from build123d import *
from OCP.BRepFilletAPI import BRepFilletAPI_MakeChamfer

# Parameters (mm, degrees)
BOSS_EXTRUDE1_DEPTH = 5
BOSS_EXTRUDE2_DEPTH = 2
SKETCH5_W           = 2.803061543
SKETCH5_H           = 5
BOSS_EXTRUDE3_DEPTH = 1
BOSS_EXTRUDE4_DEPTH = 0.5
SKETCH7_W           = 5
SKETCH7_H           = 38
CHAMFER1_SIZE       = 0.3
CHAMFER1_SIZE2      = 0.173205081


with BuildPart() as part:
    # Sketch2 → Boss-Extrude1 (new, symmetric)
    with BuildSketch(Plane.XY):
        with BuildLine():
            Line((-14.696938457, 34.5), (-14.696938457, 9.5))
            ThreePointArc((-14.696938457, 9.5), (-16.784612343, 4.952452777), (-17.5, 0))
            Line((-17.5, 0), (-40, 0))
            ThreePointArc((-40, 0), (-35.043919369, 19.285323831), (-21.403814237, 33.791666667))
            Line((-21.403814237, 33.791666667), (-21.403814237, 30.791666667))
            ThreePointArc((-21.403814237, 30.791666667), (-18.145358092, 32.817616911), (-14.696938457, 34.5))
        make_face()
    extrude(amount=BOSS_EXTRUDE1_DEPTH, both=True)

    # Sketch4 → Boss-Extrude2 (add)
    with BuildSketch(Plane.XY.offset(5)):
        Polygon((-17.5, 15), (-20, 14), (-20, 11), (-17.5, 10), (-17.5, 7), (-20, 6), (-20, 3), (-17.5, 2), (-17.5, 0), (-32.5, 0), (-32.5, 6.5), (-29.25, 9), (-29.25, 13), (-26, 15.5), (-26, 22), (-17.5, 22), align=None)
    extrude(amount=BOSS_EXTRUDE2_DEPTH)

    # Sketch5 → Boss-Extrude3 (add)
    with BuildSketch(Plane.XY.offset(5)):
        with Locations((-16.098469229, 17.5)):
            Rectangle(SKETCH5_W, SKETCH5_H)
    extrude(amount=BOSS_EXTRUDE3_DEPTH)

    # Sketch6 → Boss-Extrude4 (add)
    with BuildSketch(Plane.XY.offset(5)):
        Polygon((-26, 22), (-18.5, 26.5), (-17.5, 26.5), (-17.5, 22), align=None)
    extrude(amount=BOSS_EXTRUDE4_DEPTH)

    # Sketch7 → Cut-Revolve1 (revolve, cut)
    with BuildSketch(Plane(origin=(0, 0, 0), x_dir=(0, 0, -1), z_dir=(1, 0, 0))):
        with Locations((0, 19)):
            Rectangle(SKETCH7_W, SKETCH7_H)
    revolve(axis=Axis((0, 0, 2.5), (0, 0, -1)), mode=Mode.SUBTRACT)

    # Mirror1: part across plane


with BuildPart() as part_1:
    add(part.part)
    add(part.part.mirror(Plane.ZX))

    # Chamfer1: one chamfer whose edges measure the first distance from different faces: ONE call of the kernel's chamfer builder (chamfer() names one face for all edges)
    chamfer1_edges_1 = [part_1.edges().sort_by_distance(p)[0] for p in [
        (-17.5, -18.5, 7),
    ]]
    chamfer1_side_1 = [part_1.faces().sort_by_distance(p)[0] for p in [
        (-17.5, -20.094444444, 6.072222222),
    ]]
    chamfer1_edges_2 = [part_1.edges().sort_by_distance(p)[0] for p in [
        (-18.75, -2.5, 7),
    ]]
    chamfer1_side_2 = [part_1.faces().sort_by_distance(p)[0] for p in [
        (-18.75, -2.5, 6),
    ]]
    chamfer1_edges_3 = [part_1.edges().sort_by_distance(p)[0] for p in [
        (-20, -4.5, 7),
    ]]
    chamfer1_side_3 = [part_1.faces().sort_by_distance(p)[0] for p in [
        (-20, -4.5, 6),
    ]]
    chamfer1_edges_4 = [part_1.edges().sort_by_distance(p)[0] for p in [
        (-18.75, -6.5, 7),
    ]]
    chamfer1_side_4 = [part_1.faces().sort_by_distance(p)[0] for p in [
        (-18.75, -6.5, 6),
    ]]
    chamfer1_edges_5 = [part_1.edges().sort_by_distance(p)[0] for p in [
        (-17.5, -8.5, 7),
    ]]
    chamfer1_side_5 = [part_1.faces().sort_by_distance(p)[0] for p in [
        (-17.5, -8.5, 6),
    ]]
    chamfer1_edges_6 = [part_1.edges().sort_by_distance(p)[0] for p in [
        (-18.75, -10.5, 7),
    ]]
    chamfer1_side_6 = [part_1.faces().sort_by_distance(p)[0] for p in [
        (-18.75, -10.5, 6),
    ]]
    chamfer1_edges_7 = [part_1.edges().sort_by_distance(p)[0] for p in [
        (-20, -12.5, 7),
    ]]
    chamfer1_side_7 = [part_1.faces().sort_by_distance(p)[0] for p in [
        (-20, -12.5, 6),
    ]]
    chamfer1_edges_8 = [part_1.edges().sort_by_distance(p)[0] for p in [
        (-18.75, -14.5, 7),
    ]]
    chamfer1_side_8 = [part_1.faces().sort_by_distance(p)[0] for p in [
        (-18.75, -14.5, 6),
    ]]
    chamfer1_edges_9 = [part_1.edges().sort_by_distance(p)[0] for p in [
        (-21.75, -22, 7),
    ]]
    chamfer1_side_9 = [part_1.faces().sort_by_distance(p)[0] for p in [
        (-21.75, -22, 6.25),
    ]]
    chamfer1_edges_10 = [part_1.edges().sort_by_distance(p)[0] for p in [
        (-26, -18.75, 7),
    ]]
    chamfer1_side_10 = [part_1.faces().sort_by_distance(p)[0] for p in [
        (-26, -18.75, 6),
    ]]
    chamfer1_edges_11 = [part_1.edges().sort_by_distance(p)[0] for p in [
        (-27.625, -14.25, 7),
    ]]
    chamfer1_side_11 = [part_1.faces().sort_by_distance(p)[0] for p in [
        (-27.625, -14.25, 6),
    ]]
    chamfer1_edges_12 = [part_1.edges().sort_by_distance(p)[0] for p in [
        (-29.25, -11, 7),
    ]]
    chamfer1_side_12 = [part_1.faces().sort_by_distance(p)[0] for p in [
        (-29.25, -11, 6),
    ]]
    chamfer1_edges_13 = [part_1.edges().sort_by_distance(p)[0] for p in [
        (-30.875, -7.75, 7),
    ]]
    chamfer1_side_13 = [part_1.faces().sort_by_distance(p)[0] for p in [
        (-30.875, -7.75, 6),
    ]]
    chamfer1_edges_14 = [part_1.edges().sort_by_distance(p)[0] for p in [
        (-17.5, 0, 7),
    ]]
    chamfer1_side_14 = [part_1.faces().sort_by_distance(p)[0] for p in [
        (-17.5, 0, 6),
    ]]
    chamfer1_edges_15 = [part_1.edges().sort_by_distance(p)[0] for p in [
        (-18.75, 2.5, 7),
    ]]
    chamfer1_side_15 = [part_1.faces().sort_by_distance(p)[0] for p in [
        (-18.75, 2.5, 6),
    ]]
    chamfer1_edges_16 = [part_1.edges().sort_by_distance(p)[0] for p in [
        (-20, 4.5, 7),
    ]]
    chamfer1_side_16 = [part_1.faces().sort_by_distance(p)[0] for p in [
        (-20, 4.5, 6),
    ]]
    chamfer1_edges_17 = [part_1.edges().sort_by_distance(p)[0] for p in [
        (-18.75, 6.5, 7),
    ]]
    chamfer1_side_17 = [part_1.faces().sort_by_distance(p)[0] for p in [
        (-18.75, 6.5, 6),
    ]]
    chamfer1_edges_18 = [part_1.edges().sort_by_distance(p)[0] for p in [
        (-17.5, 8.5, 7),
    ]]
    chamfer1_side_18 = [part_1.faces().sort_by_distance(p)[0] for p in [
        (-17.5, 8.5, 6),
    ]]
    chamfer1_edges_19 = [part_1.edges().sort_by_distance(p)[0] for p in [
        (-18.75, 10.5, 7),
    ]]
    chamfer1_side_19 = [part_1.faces().sort_by_distance(p)[0] for p in [
        (-18.75, 10.5, 6),
    ]]
    chamfer1_edges_20 = [part_1.edges().sort_by_distance(p)[0] for p in [
        (-20, 12.5, 7),
    ]]
    chamfer1_side_20 = [part_1.faces().sort_by_distance(p)[0] for p in [
        (-20, 12.5, 6),
    ]]
    chamfer1_edges_21 = [part_1.edges().sort_by_distance(p)[0] for p in [
        (-18.75, 14.5, 7),
    ]]
    chamfer1_side_21 = [part_1.faces().sort_by_distance(p)[0] for p in [
        (-18.75, 14.5, 6),
    ]]
    chamfer1_edges_22 = [part_1.edges().sort_by_distance(p)[0] for p in [
        (-17.5, 18.5, 7),
    ]]
    chamfer1_side_22 = [part_1.faces().sort_by_distance(p)[0] for p in [
        (-17.5, 20.094444444, 6.072222222),
    ]]
    chamfer1_edges_23 = [part_1.edges().sort_by_distance(p)[0] for p in [
        (-21.75, 22, 7),
    ]]
    chamfer1_side_23 = [part_1.faces().sort_by_distance(p)[0] for p in [
        (-21.75, 22, 6.25),
    ]]
    chamfer1_edges_24 = [part_1.edges().sort_by_distance(p)[0] for p in [
        (-26, 18.75, 7),
    ]]
    chamfer1_side_24 = [part_1.faces().sort_by_distance(p)[0] for p in [
        (-26, 18.75, 6),
    ]]
    chamfer1_edges_25 = [part_1.edges().sort_by_distance(p)[0] for p in [
        (-27.625, 14.25, 7),
    ]]
    chamfer1_side_25 = [part_1.faces().sort_by_distance(p)[0] for p in [
        (-27.625, 14.25, 6),
    ]]
    chamfer1_edges_26 = [part_1.edges().sort_by_distance(p)[0] for p in [
        (-29.25, 11, 7),
    ]]
    chamfer1_side_26 = [part_1.faces().sort_by_distance(p)[0] for p in [
        (-29.25, 11, 6),
    ]]
    chamfer1_edges_27 = [part_1.edges().sort_by_distance(p)[0] for p in [
        (-30.875, 7.75, 7),
    ]]
    chamfer1_side_27 = [part_1.faces().sort_by_distance(p)[0] for p in [
        (-30.875, 7.75, 6),
    ]]
    chamfer1_edges_28 = [part_1.edges().sort_by_distance(p)[0] for p in [
        (-32.5, 0, 7),
    ]]
    chamfer1_side_28 = [part_1.faces().sort_by_distance(p)[0] for p in [
        (-32.5, 0, 6),
    ]]
    chamfer1 = BRepFilletAPI_MakeChamfer(part_1.part.solid().wrapped)
    for e in chamfer1_edges_1:
        chamfer1.Add(CHAMFER1_SIZE, CHAMFER1_SIZE2, e.wrapped, chamfer1_side_1[0].wrapped)  # the first distance lies on this face
    for e in chamfer1_edges_2:
        chamfer1.Add(CHAMFER1_SIZE, CHAMFER1_SIZE2, e.wrapped, chamfer1_side_2[0].wrapped)  # the first distance lies on this face
    for e in chamfer1_edges_3:
        chamfer1.Add(CHAMFER1_SIZE, CHAMFER1_SIZE2, e.wrapped, chamfer1_side_3[0].wrapped)  # the first distance lies on this face
    for e in chamfer1_edges_4:
        chamfer1.Add(CHAMFER1_SIZE, CHAMFER1_SIZE2, e.wrapped, chamfer1_side_4[0].wrapped)  # the first distance lies on this face
    for e in chamfer1_edges_5:
        chamfer1.Add(CHAMFER1_SIZE, CHAMFER1_SIZE2, e.wrapped, chamfer1_side_5[0].wrapped)  # the first distance lies on this face
    for e in chamfer1_edges_6:
        chamfer1.Add(CHAMFER1_SIZE, CHAMFER1_SIZE2, e.wrapped, chamfer1_side_6[0].wrapped)  # the first distance lies on this face
    for e in chamfer1_edges_7:
        chamfer1.Add(CHAMFER1_SIZE, CHAMFER1_SIZE2, e.wrapped, chamfer1_side_7[0].wrapped)  # the first distance lies on this face
    for e in chamfer1_edges_8:
        chamfer1.Add(CHAMFER1_SIZE, CHAMFER1_SIZE2, e.wrapped, chamfer1_side_8[0].wrapped)  # the first distance lies on this face
    for e in chamfer1_edges_9:
        chamfer1.Add(CHAMFER1_SIZE, CHAMFER1_SIZE2, e.wrapped, chamfer1_side_9[0].wrapped)  # the first distance lies on this face
    for e in chamfer1_edges_10:
        chamfer1.Add(CHAMFER1_SIZE, CHAMFER1_SIZE2, e.wrapped, chamfer1_side_10[0].wrapped)  # the first distance lies on this face
    for e in chamfer1_edges_11:
        chamfer1.Add(CHAMFER1_SIZE, CHAMFER1_SIZE2, e.wrapped, chamfer1_side_11[0].wrapped)  # the first distance lies on this face
    for e in chamfer1_edges_12:
        chamfer1.Add(CHAMFER1_SIZE, CHAMFER1_SIZE2, e.wrapped, chamfer1_side_12[0].wrapped)  # the first distance lies on this face
    for e in chamfer1_edges_13:
        chamfer1.Add(CHAMFER1_SIZE, CHAMFER1_SIZE2, e.wrapped, chamfer1_side_13[0].wrapped)  # the first distance lies on this face
    for e in chamfer1_edges_14:
        chamfer1.Add(CHAMFER1_SIZE, CHAMFER1_SIZE2, e.wrapped, chamfer1_side_14[0].wrapped)  # the first distance lies on this face
    for e in chamfer1_edges_15:
        chamfer1.Add(CHAMFER1_SIZE, CHAMFER1_SIZE2, e.wrapped, chamfer1_side_15[0].wrapped)  # the first distance lies on this face
    for e in chamfer1_edges_16:
        chamfer1.Add(CHAMFER1_SIZE, CHAMFER1_SIZE2, e.wrapped, chamfer1_side_16[0].wrapped)  # the first distance lies on this face
    for e in chamfer1_edges_17:
        chamfer1.Add(CHAMFER1_SIZE, CHAMFER1_SIZE2, e.wrapped, chamfer1_side_17[0].wrapped)  # the first distance lies on this face
    for e in chamfer1_edges_18:
        chamfer1.Add(CHAMFER1_SIZE, CHAMFER1_SIZE2, e.wrapped, chamfer1_side_18[0].wrapped)  # the first distance lies on this face
    for e in chamfer1_edges_19:
        chamfer1.Add(CHAMFER1_SIZE, CHAMFER1_SIZE2, e.wrapped, chamfer1_side_19[0].wrapped)  # the first distance lies on this face
    for e in chamfer1_edges_20:
        chamfer1.Add(CHAMFER1_SIZE, CHAMFER1_SIZE2, e.wrapped, chamfer1_side_20[0].wrapped)  # the first distance lies on this face
    for e in chamfer1_edges_21:
        chamfer1.Add(CHAMFER1_SIZE, CHAMFER1_SIZE2, e.wrapped, chamfer1_side_21[0].wrapped)  # the first distance lies on this face
    for e in chamfer1_edges_22:
        chamfer1.Add(CHAMFER1_SIZE, CHAMFER1_SIZE2, e.wrapped, chamfer1_side_22[0].wrapped)  # the first distance lies on this face
    for e in chamfer1_edges_23:
        chamfer1.Add(CHAMFER1_SIZE, CHAMFER1_SIZE2, e.wrapped, chamfer1_side_23[0].wrapped)  # the first distance lies on this face
    for e in chamfer1_edges_24:
        chamfer1.Add(CHAMFER1_SIZE, CHAMFER1_SIZE2, e.wrapped, chamfer1_side_24[0].wrapped)  # the first distance lies on this face
    for e in chamfer1_edges_25:
        chamfer1.Add(CHAMFER1_SIZE, CHAMFER1_SIZE2, e.wrapped, chamfer1_side_25[0].wrapped)  # the first distance lies on this face
    for e in chamfer1_edges_26:
        chamfer1.Add(CHAMFER1_SIZE, CHAMFER1_SIZE2, e.wrapped, chamfer1_side_26[0].wrapped)  # the first distance lies on this face
    for e in chamfer1_edges_27:
        chamfer1.Add(CHAMFER1_SIZE, CHAMFER1_SIZE2, e.wrapped, chamfer1_side_27[0].wrapped)  # the first distance lies on this face
    for e in chamfer1_edges_28:
        chamfer1.Add(CHAMFER1_SIZE, CHAMFER1_SIZE2, e.wrapped, chamfer1_side_28[0].wrapped)  # the first distance lies on this face
    add(Compound.cast(chamfer1.Shape()), mode=Mode.REPLACE)


solid = part_1.part
Model file for the job. Use its own axes, mm. A direction names the side the tool comes from. Round coordinates to 2 decimals unless told otherwise and drop trailing zeros. Loops run counter-clockwise (first coordinate to the right, second up) from the corner with the lowest first, then second, coordinate; pieces in that order, holes last.
1. Band-saw the part on B-B, the plane x = -31. List the corners of the cut face in (y, z), and give its area (3 significant figures).
Check values:
outline: (-25.28, -5) - (25.28, -5) - (25.28, 5) - (7.65, 5) - (7.65, 6.7) - (7.44, 7) - (-7.44, 7) - (-7.65, 6.7) - (-7.65, 5) - (-25.28, 5) - close; hole (-21.98, -2.5) - (21.98, -2.5) - (21.98, 2.5) - (-21.98, 2.5) - close
area: 316 mm2
2. Tool access for faces 4 (the flat face through (-17.5, 9, 6)), 5 (the flat face through (-24, 0, -2.5)), 6 (the flat face through (-32.5, 0, 6)), 7 (the flat face through (-27.65, -14.23, 5.84)), 8 (the flat face through (-14.697, 22, -4)): list every direction of +Z, -Z, +X, -X, +Y, -Y with a clear straight run to the whole face (end or side of a thin tool).
Check values:
face 4: +Z, +X
face 5: +X
face 6: +Z, -X, +Y, -Y
face 7: +Z, -X, -Y
face 8: +Z, -Z, +X, +Y, -Y
3. Drop flat-ended pins along their axis: P1, Ø3, axis at y = 4, z = 4, coming from the -X side; P2, Ø5, axis at x = -29.5, y = 13.5, coming from the +Z side; P3, Ø1.9, axis at y = 11, z = 5.5, coming from the -X side; P4, Ø1.4, axis at x = -15.5, y = 17, coming from the +Z side. Give the stop position or say it passes through.
Check values:
P1: stops at x = -39.92
P2: stops at z = 7
P3: stops at x = -38.68
P4: stops at z = 6
4. Band-saw the part on C-C, the plane x = -16.75. List the corners of the cut face in (y, z).
Check values:
outline: (-33.55, -5) - (-5.07, -5) - (-5.07, -2.5) - (-33.55, -2.5) - close; (-33.55, 2.5) - (-5.07, 2.5) - (-5.07, 5) - (-15, 5) - (-15, 6) - (-20, 6) - (-20, 5) - (-33.55, 5) - close; (5.07, -5) - (33.55, -5) - (33.55, -2.5) - (5.07, -2.5) - close; (5.07, 2.5) - (33.55, 2.5) - (33.55, 5) - (20, 5) - (20, 6) - (15, 6) - (15, 5) - (5.07, 5) - close
5. Band-saw the part on D-D, the plane y = -12. List the corners of the cut face in (x, z).
Check values:
outline: (-38.16, -5) - (-14.7, -5) - (-14.7, -2.5) - (-36.06, -2.5) - (-36.06, 2.5) - (-14.7, 2.5) - (-14.7, 5) - (-20, 5) - (-20, 6.7) - (-20.17, 7) - (-29.08, 7) - (-29.25, 6.7) - (-29.25, 5) - (-38.16, 5) - close
6. Wall check: probe 1 along Z at (x, y) = (-23, 0); probe 2 along Z at (x, y) = (-16.5, -8.5); probe 3 along X at (y, z) = (13, 5.25). Give the ranges that are in metal, low to high.
Check values:
probe 1: z = -5 to -2.5, 2.5 to 7
probe 2: z = -5 to -2.5, 2.5 to 5
probe 3: x = -29.25 to -20
7. Band-saw the part on A-A, the plane z = -3.75. List the corners of the cut face in (x, y).
Check values:
outline: (-21.4, -33.79) - (-21.4, -30.79) arc R37.5 ccw to (-14.7, -34.5) - (-14.7, -9.5) arc R17.5 cw to (-14.7, 9.5) - (-14.7, 34.5) arc R37.5 ccw to (-21.4, 30.79) - (-21.4, 33.79) arc R40 ccw to start
8. Mould opens along X. For faces 1 (the cylindrical face through (-18.192, -32.792, -3.732)), 2 (the flat face through (-20, 13, 6)), 3 (the flat face through (-24, 0, 2.5)) say: +X half, -X half, draft (parallel to the pull), parting line (faces both ways), or undercut.
Check values:
face 1: undercut
face 2: +X half
face 3: draft
